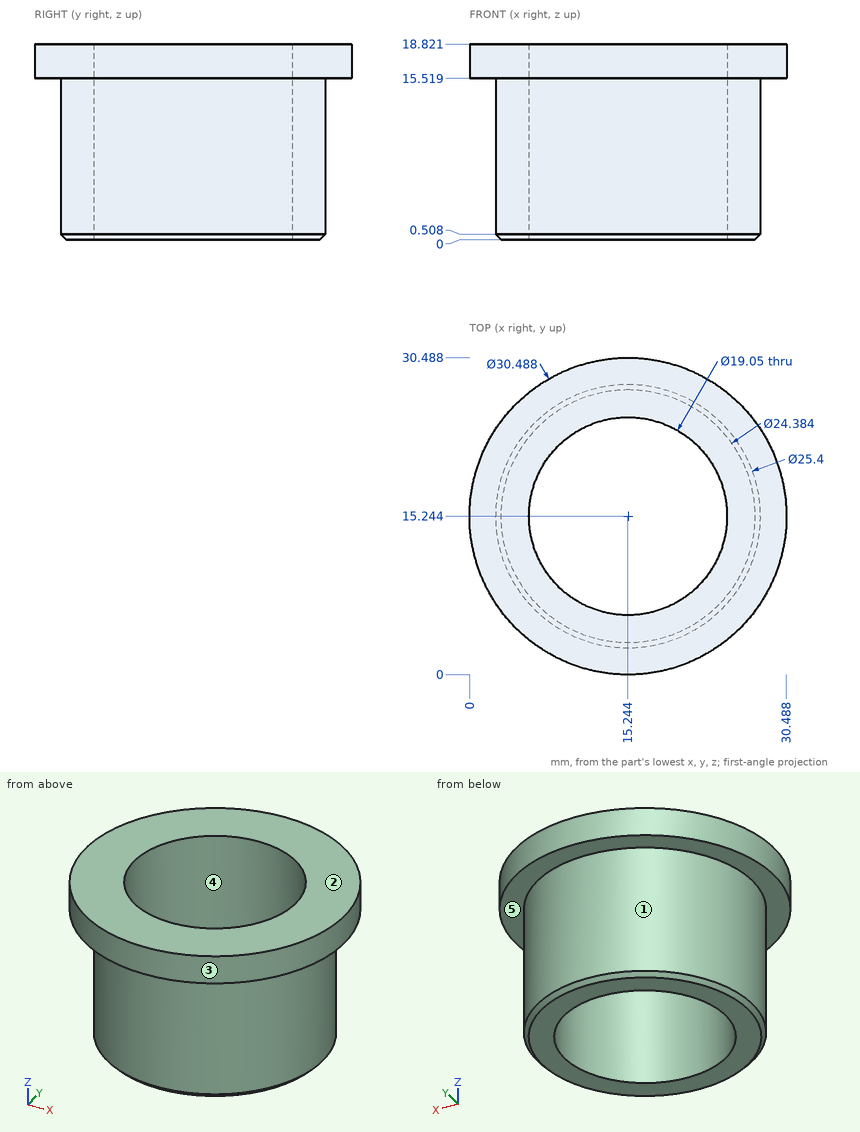
Print and shaded views of the part. All mm, measured from the part's lowest x, y and z. A direction names the side the tool comes from. Coordinates: 2 decimals unless noted, no trailing zeros. Use CSV: the item, a comma, the result in double quotes. Start each with the question number.
Q1. 3-axis set-ups, long thin cutter, end or side, ignore diameter. For the marked faces 1 and 2: which of +Z, -Z, +X, -X, +Y, -Y reach the whole face in a straight line?
Q2. Flat gauge pins, fed straight in: pin 1 Ø5 at (x, z) = (17, 9.5) entering from -Y; pin 2 Ø3 at (x, z) = (5, 16.5) entering from +Y; pin 3 Ø4 at (x, z) = (22, 10) entering from -Y. Where does each tip first touch, or does it go through?
Q3. Drill centre lines: probe 1 along Z at (x, y) = (2, 18); probe 2 along Y at (x, z) = (18, 7.5); probe 3 along Y at (x, z) = (19.5, 10) (1 decimal). Where is each one in solid material? Low to high.
Q4. Pull direction Y, two halves, no side cores. Call the marked faces 3, 4 and 5: released by +Y, released by -Y, zero draft, split by the parting line, or undercut.
Checked values:
1,face 1,"-Z"
1,face 2,"+Z, +X, -X, +Y, -Y"
2,pin 1,"stops at y = 2.54"
2,pin 2,"stops at y = 27.73"
2,pin 3,"stops at y = 3.47"
3,probe 1,"z = 15.52 to 18.82"
3,probe 2,"y = 2.85 to 6.13, 24.36 to 27.64"
3,probe 3,"y = 3.3 to 6.7, 23.8 to 27.2"
4,face 3,"split by the parting line"
4,face 4,"undercut"
4,face 5,"zero draft"
